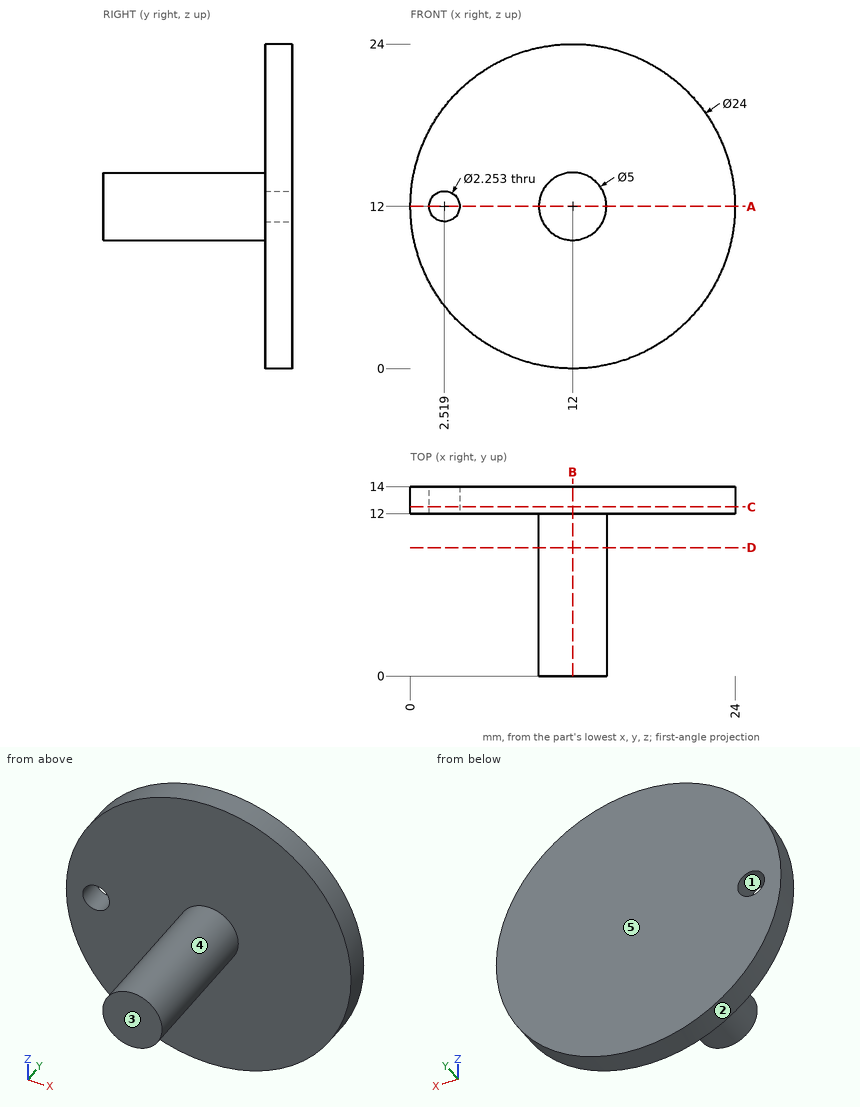
Study the drawing (mm; zero at the part's minimum x, y, z) and answer. A direction names the side the tool comes from. Give positions to 0.01 mm unless a question says otherwise; leave off trailing zeros. Write each loop counter-clockwise with the first axis right and the second up, starting at its lowest first coordinate (ties: lowest second). Pieces come first, ordered by that corner, then holes.
Item 1: Flat-ended cylindrical pins translate along their axes: P1, Ø1.5, axis at x = 13.5, y = 2.5, coming from the +Z side (1 decimal); P2, Ø8, axis at y = 10.5, z = 21.5, coming from the -X side; P3, Ø3.5, axis at x = 2.52, z = 12, coming from the -Y side; P4, Ø12, axis at x = 11, z = 9, coming from the -Y side. Find the tip coordinate at first contact, or state that the pin passes through.
Item 2: Section B-B, the plane x = 12 is taken. Write down the section's boundary in (y, z).
Item 3: Section D-D, the plane y = 9.5 is taken. Write down the section's boundary in (x, z).
Item 4: Section A-A, the plane z = 12 is taken. Write down the section's boundary in (x, y) (1 decimal), plus the area to 4 significant figures.
Item 5: Which of the six approach directions +Z, -Z, +X, -X, +Y, -Y give full straight-line access (tool end or side, diameter ignored) to the marked faces 4 and 5?
Item 6: Find the intervals of material crossed by line 1 along Y through (x, z) = (21, 9.25); line 2 along Z through (x, y) = (12, 9.25); line 3 along Z through (x, y) = (11.25, 10.5) (1 decimal), in increasing order.
Item 7: Determine the mould class of the marked faces 1, 2 and 3 for opening direction X: released by +X, released by -X, zero draft, split by the parting line, or undercut.
Item 8: Section C-C, the plane y = 12.5 is taken. Write down the section's boundary in (x, z) (1 decimal).
Completed:
1. P1: stops at z = 14.4
1. P2: stops at x = 1.49
1. P3: stops at y = 12
1. P4: stops at y = 0
2. outline: (0, 9.5) - (12, 9.5) - (12, 0) - (14, 0) - (14, 24) - (12, 24) - (12, 14.5) - (0, 14.5) - close
3. outline: circle Ø5 at (12, 12)
4. outline: (0, 12) - (1.4, 12) - (1.4, 14) - (0, 14) - close; (3.6, 12) - (9.5, 12) - (9.5, 0) - (14.5, 0) - (14.5, 12) - (24, 12) - (24, 14) - (3.6, 14) - close
4. area: 103.5 mm2
5. face 4: -Y
5. face 5: +Z, -Z, +X, -X, +Y
6. line 1: y = 12 to 14
6. line 2: z = 9.5 to 14.5
6. line 3: z = 9.6 to 14.4
7. face 1: undercut
7. face 2: split by the parting line
7. face 3: zero draft
8. outline: circle Ø24 at (12, 12); hole circle Ø2.3 at (2.5, 12)
